Could you check a few things on this model? Use its own coordinates, in mm. Face numbers are marked on the shaded views. A direction names the side the tool comes from. Round coordinates to 2 decimals unless told otherwise and drop trailing zeros. Order: outer loops, then holes, each group sorted by start corner. A loop starts at its lowest first (then second) coordinate and runs counter-clockwise, first axis right, second up. Notation, with made-up numbers: M 89.25,-4 L 94.25,-4 A20 ccw 94.25,24 Z; hole C -14,-37.75 d5. An arc over 180 degrees is marked long. Write each question's results on one line, items separated by ' | '. Start each with the question number.
1. For the marked faces 1, 2 and 3, which set-ups out of +Z, -Z, +X, -X, +Y, -Y let a thin tool reach every point of the face, with its end or its side?
2. Suppose I cut it at B-B on z = 0. Write out the boundary of the cut face in (x, y).
3. I'm going to push flat-ended pins straight in: pin 1 (6 mm diameter, centred on x = -59, y = 0, fed in from -Z); pin 2 (1 mm diameter, centred on y = 33.5, z = 2, fed in from -X); pin 3 (2 mm diameter, centred on y = 1, z = 2, fed in from +X); pin 4 (4 mm diameter, centred on x = 1.5, z = -1, fed in from +Y). Where does each tip first touch, or does it pass through?
4. Please list where these lines run through material, in increasing order: L1, parallel to Y at x = -59, z = 2.5; L2, parallel to Y at x = -43, z = 0.5; L3, parallel to Y at x = 11.5, z = 4.
5. Suppose I cut it at A-A on y = 0. Write out the boundary of the cut face in (x, z), and give its area (3 significant figures).
6. Suppose I cut it at D-D on x = -4. Write out the boundary of the cut face in (y, z).
7. Suppose I cut it at C-C on x = -34.5. Write out the boundary of the cut face in (y, z), and give its area (3 significant figures).
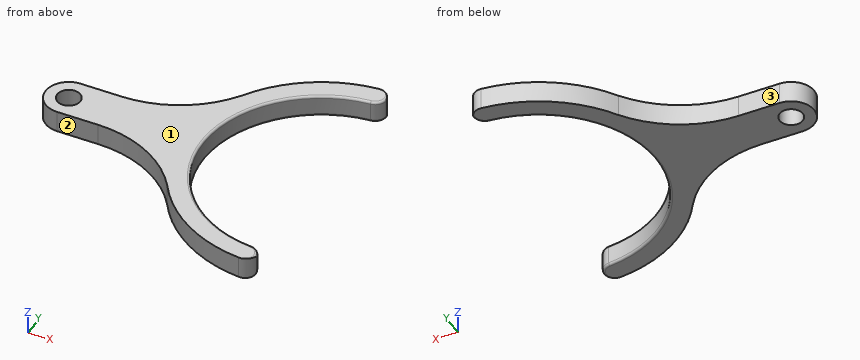
from build123d import *

# Parameters (mm, degrees)
SKETCH1_R           = 5.02
BOSS_EXTRUDE1_DEPTH = 4.75
FILLET2_R           = 5
FILLET3_R           = 1


with BuildPart() as part:
    # Sketch1 → Boss-Extrude1 (new, symmetric)
    with BuildSketch(Plane.XY):
        with BuildLine():
            Line((51, -60), (51, -51))
            ThreePointArc((51, -51), (0, 0), (51, 51))
            Line((51, 51), (51, 60))
            ThreePointArc((51, 60), (21.814538512, 52.423361565), (0, 31.606961259))
            ThreePointArc((0, 31.606961259), (-17.914586674, 15.730078286), (-41.156231011, 10))
            Line((-41.156231011, 10), (-59, 10))
            ThreePointArc((-59, 10), (-69, 0), (-59, -10))
            Line((-59, -10), (-41.156231011, -10))
            ThreePointArc((-41.156231011, -10), (-17.914586674, -15.730078286), (0, -31.606961259))
            ThreePointArc((0, -31.606961259), (21.814538512, -52.423361565), (51, -60))
        make_face()
        with Locations((-59, 0)):
            Circle(SKETCH1_R, mode=Mode.SUBTRACT)
    extrude(amount=BOSS_EXTRUDE1_DEPTH, both=True)

    # Fillet2
    # the kernel refuses this fillet: 5 mm, written as the material it takes off along each edge
    with BuildSketch(Plane(origin=(51, -60, 18.400501973), x_dir=(0, 1, 0), z_dir=(0, 0, -1))) as fillet2_piece_1:
        with BuildLine():
            CenterArc((5.227744249, -5), FILLET2_R, 90, 95.21590857)
            ThreePointArc((0.248448272, -5.454545455), (0.062144251, -2.730100395), (0, 0))
            Line((0, 0), (5.227744249, 0))
        make_face()
    extrude(amount=36.801003947, mode=Mode.SUBTRACT)
    with BuildSketch(Plane(origin=(51, -51, -16.690847674), x_dir=(0, -1, 0), z_dir=(0, 0, 1))) as fillet2_piece_2:
        with BuildLine():
            CenterArc((4.77633907, -5), FILLET2_R, 90, 84.8774839)
            ThreePointArc((-0.203691205, -4.553571429), (-0.050948249, -2.279062464), (0, 0))
            Line((0, 0), (4.77633907, 0))
        make_face()
    extrude(amount=33.381695348, mode=Mode.SUBTRACT)
    with BuildSketch(Plane(origin=(51, 60, -18.400501973), x_dir=(-0.9989642624898897, -0.04550167324429649, 0), z_dir=(0, 0, 1))) as fillet2_piece_3:
        with BuildLine():
            CenterArc((5.232692423, 4.994821312), FILLET2_R, 177.392045715, 95.21590857)
            Line((0.237871111, 5.222329679), (0, 0))
            ThreePointArc((0, 0), (2.730100395, -0.062144251), (5.460200789, 0))
        make_face()
    extrude(amount=36.801003947, mode=Mode.SUBTRACT)
    with BuildSketch(Plane(origin=(51, 51, -16.690847674), x_dir=(0, 1, 0), z_dir=(0, 0, 1))) as fillet2_piece_4:
        with BuildLine():
            CenterArc((4.77633907, 5), FILLET2_R, 185.1225161, 84.8774839)
            ThreePointArc((-0.203691205, 4.553571429), (-0.050948249, 2.279062464), (0, 0))
            Line((0, 0), (4.77633907, 0))
        make_face()
    extrude(amount=33.381695348, mode=Mode.SUBTRACT)

    # Fillet3
    fillet3_edges = [part.edges().sort_by_distance(p)[0] for p in [
        (0, 0, -4.75),
        (49.515727495, 52.221109094, -4.75),
        (49.515727495, -52.221109094, -4.75),
        (0, 0, 4.75),
        (49.515727495, 52.221109094, 4.75),
        (49.515727495, -52.221109094, 4.75),
    ]]
    fillet(fillet3_edges, radius=FILLET3_R)


solid = part.part
Filled sheet:
1) face 1: +Z, +X, -X, +Y, -Y | face 2: +Z, -Z, -X, -Y | face 3: +Z, -Z, -X, +Y
2) outline: M -59,-10 L -41.16,-10 A50 cw 0,-31.61 A60 ccw 45.55,-59.75 A5 ccw 50.97,-55.27 A5 ccw 46.45,-50.8 A51 cw 46.45,50.8 A5 ccw 50.97,55.27 A5 ccw 45.55,59.75 A60 ccw 0,31.61 A50 cw -41.16,10 L -59,10 A10 ccw Z; hole C -59,0 d10.04
3) pin 1: passes through | pin 2: stops at x = 0.89 | pin 3: stops at x = 0.04 | pin 4: stops at y = 36.66
4) L1: y = -10 to -5.02, 5.02 to 10 | L2: y = -10 to 10 | L3: y = -45.16 to -32.31, 32.31 to 45.16
5) outline: M -69,-4.75 L -64.02,-4.75 L -64.02,4.75 L -69,4.75 Z; M -53.98,-4.75 L -1,-4.75 A1 ccw 0,-3.75 L 0,3.75 A1 ccw -1,4.75 L -53.98,4.75 Z | area: 560 mm^2
6) outline: M -26.54,-4.75 L 26.54,-4.75 L 26.54,4.75 L -26.54,4.75 Z
7) outline: M -10.45,-4.75 L 10.45,-4.75 L 10.45,4.75 L -10.45,4.75 Z | area: 198 mm^2
